The model under review builds one solid part; all positions refer to its coordinate system, in mm. Face numbers are marked on the shaded views. Coordinates: 2 decimals unless noted, no trailing zeros. Write each loop counter-clockwise with the first axis right and the second up, starting at its lowest first coordinate (ties: lowest second). Pieces come first, ordered by that corner, then holes. Notation, with made-up numbers: (57.25, 53.5) - (101.25, 53.5) arc R29 cw to (101.25, 77.5) - close; hole circle Ø3 at (21.25, -25). An arc over 180 degrees is marked (long way). Return JSON: item names as keys, results as strings. Group by question number.
(1) We need section C-C on z = 1.3. State the section outline as (x, y) points.
(2) Draft analysis for pull direction X (two halves, no side actions). For the marked faces 1 and 2, state which applies: released by +X, released by -X, zero draft, split by the parting line, or undercut.
(3) To check wall thickness, follow L1, parallel to Y at x = 13, z = 2.3; L2, parallel to Y at x = 13, z = 1.25; L3, parallel to Y at x = 0, z = 1.15. State the ranges of each line that lie inside material, in increasing order. Write a range as from..to.
(4) We need section A-A on y = -33. State the section outline as (x, z) points, then the cut area to 3 significant figures.
(5) We need section D-D on x = 0. State the section outline as (y, z) points.
(6) For pin 1 Ø6 at (x, y) = (-11.5, 8.5) entering from -Z; pin 2 Ø17 at (x, y) = (4, -12.5) entering from -Z; pin 3 Ø21.5 at (x, y) = (0, 0) entering from -Z, all flat-tipped, find the tip position at first contact; note any pin that passes through.
(7) We need section B-B on x = 13. State the section outline as (y, z) points, then the cut area to 3 significant figures.
```python
from build123d import *

# Parameters (mm, degrees)
ESQUISSE1_W             = 34
ESQUISSE1_H             = 74
BOSS_EXTRU_1_DEPTH      = 2
ESQUISSE2_W             = 32
ESQUISSE2_H             = 70
BOSS_EXTRU_2_DEPTH      = 2
SKETCH1_R               = 6.75
CUT_EXTRUDE1_DEPTH      = 41.914545091
ESQUISSE3_R             = 1
ENL_V_MAT_EXTRU_1_DEPTH = 41.914545091
ESQUISSE4_W             = 10
ESQUISSE4_H             = 10
BOSS_EXTRU_3_DEPTH      = 2
CONG_1_R                = 2


with BuildPart() as part:
    # Esquisse1 → Boss.-Extru.1 (new body)
    with BuildSketch(Plane.XY):
        Rectangle(ESQUISSE1_W, ESQUISSE1_H)
    extrude(amount=BOSS_EXTRU_1_DEPTH)

    # Esquisse2 → Boss.-Extru.2 (add)
    with BuildSketch(Plane.XY.offset(2)):
        with Locations((-1, 0)):
            Rectangle(ESQUISSE2_W, ESQUISSE2_H)
    extrude(amount=BOSS_EXTRU_2_DEPTH)

    # Sketch1 → Cut-Extrude1 (cut, through all)
    with BuildSketch(Plane(origin=(0, 0, 0), x_dir=(-1, 0, 0), z_dir=(0, 0, -1))):
        Circle(SKETCH1_R)
    extrude(amount=-CUT_EXTRUDE1_DEPTH, mode=Mode.SUBTRACT)

    # Esquisse3 → Enlèv. mat.-Extru.1 (cut, through all)
    with BuildSketch(Plane.XY.offset(4)):
        with Locations((-15, 33)):
            Circle(ESQUISSE3_R)
        with Locations((13, 33)):
            Circle(ESQUISSE3_R)
        with Locations((13, -33)):
            Circle(ESQUISSE3_R)
        with Locations((-15, -33)):
            Circle(ESQUISSE3_R)
    extrude(amount=-ENL_V_MAT_EXTRU_1_DEPTH, mode=Mode.SUBTRACT)

    # Esquisse4 → Boss.-Extru.3 (add)
    with BuildSketch(Plane(origin=(0, 0, 0), x_dir=(-1, 0, 0), z_dir=(0, 0, -1))):
        with Locations((16, 0)):
            Rectangle(ESQUISSE4_W, ESQUISSE4_H)
    extrude(amount=BOSS_EXTRU_3_DEPTH)

    # Congé1
    cong_1_edges = [part.edges().sort_by_distance(p)[0] for p in [
        (-14, -5, 0),
        (-11, 0, 0),
        (-14, 5, 0),
        (-21, 5, -1),
        (-21, -5, -1),
    ]]
    fillet(cong_1_edges, radius=CONG_1_R - 0.0001)  # a hair under: the kernel refuses the full size


solid = part.part
```
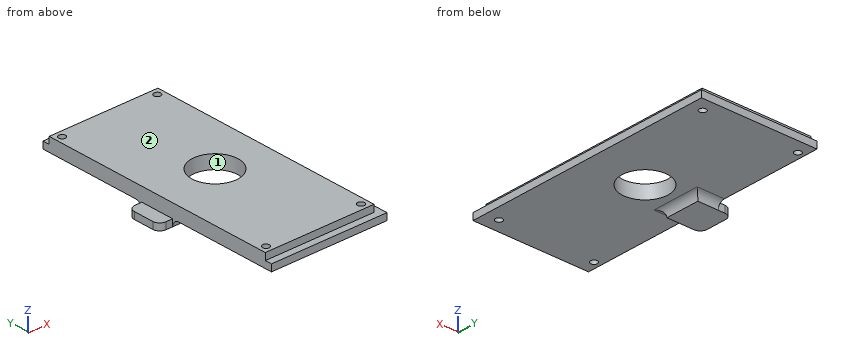
Ans:
{
 "1": {"outline": "(-17, -37) - (17, -37) - (17, 37) - (-17, 37) - close; hole circle Ø2 at (-15, -33); hole circle Ø2 at (-15, 33); hole circle Ø13.5 at (0, 0); hole circle Ø2 at (13, -33); hole circle Ø2 at (13, 33)"},
 "2": {"face 1": "undercut", "face 2": "zero draft"},
 "3": {"L1": "-35..-34, -32..32, 34..35", "L2": "-37..-34, -32..32, 34..37", "L3": "-37..-6.75, 6.75..37"},
 "4": {"outline": "(-17, 0) - (-16, 0) - (-16, 4) - (-17, 4) - close; (-14, 0) - (12, 0) - (12, 4) - (-14, 4) - close; (14, 0) - (17, 0) - (17, 2) - (15, 2) - (15, 4) - (14, 4) - close", "area": "116 mm²"},
 "5": {"outline": "(-37, 0) - (-6.75, 0) - (-6.75, 4) - (-35, 4) - (-35, 2) - (-37, 2) - close; (6.75, 0) - (37, 0) - (37, 2) - (35, 2) - (35, 4) - (6.75, 4) - close"},
 "6": {"pin 1": "z = -0.68", "pin 2": "z = 0", "pin 3": "z = -1.03"},
 "7": {"outline": "(-37, 0) - (-34, 0) - (-34, 4) - (-35, 4) - (-35, 2) - (-37, 2) - close; (-32, 0) - (32, 0) - (32, 4) - (-32, 4) - close; (34, 0) - (37, 0) - (37, 2) - (35, 2) - (35, 4) - (34, 4) - close", "area": "272 mm²"}
}
